Check sheet for the modelled part. Datum: model origin and axes. Units: mm. Face numbers are marked on the shaded views. A direction names the side the tool comes from. Give positions to 0.01 mm unless a question says otherwise; leave off trailing zeros. Order: outer loops, then holes, each group sorted by start corner. A loop starts at its lowest first (then second) coordinate and runs counter-clockwise, first axis right, second up.
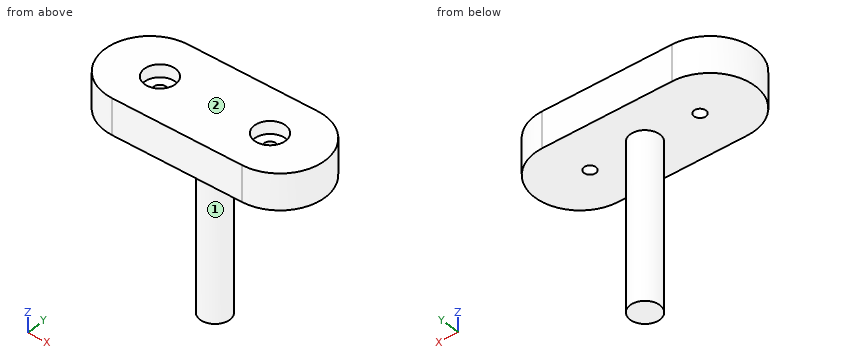
```python
from build123d import *

# Parameters (mm, degrees)
SALIENTE_EXTRUIR1_DEPTH = 9.63
CROQUIS2_R              = 3.98
SALIENTE_EXTRUIR2_DEPTH = 44.5
CROQUIS3_R              = 1.6
CORTAR_EXTRUIR1_DEPTH   = 63.977202423
CROQUIS4_R              = 4.18
CORTAR_EXTRUIR2_DEPTH   = 3.39


with BuildPart() as part:
    # Croquis1 → Saliente-Extruir1 (new body)
    with BuildSketch(Plane.XY):
        with BuildLine():
            Line((-17.685, 12.13), (17.685, 12.13))
            ThreePointArc((17.685, 12.13), (29.815, 0), (17.685, -12.13))
            Line((17.685, -12.13), (-17.685, -12.13))
            ThreePointArc((-17.685, -12.13), (-29.815, 0), (-17.685, 12.13))
        make_face()
    extrude(amount=-SALIENTE_EXTRUIR1_DEPTH)

    # Croquis2 → Saliente-Extruir2 (add)
    with BuildSketch(Plane(origin=(0, 0, -9.63), x_dir=(-1, 0, 0), z_dir=(0, 0, -1))):
        with Locations(Location((0, 0, 0), (0, 0, 180))):
            Circle(CROQUIS2_R)
    extrude(amount=SALIENTE_EXTRUIR2_DEPTH)

    # Croquis3 → Cortar-Extruir1 (cut, through all)
    with BuildSketch(Plane.XY):
        with Locations((-15, 0)):
            Circle(CROQUIS3_R)
        with Locations((15, 0)):
            Circle(CROQUIS3_R)
    extrude(amount=-CORTAR_EXTRUIR1_DEPTH, mode=Mode.SUBTRACT)

    # Croquis4 → Cortar-Extruir2 (cut)
    with BuildSketch(Plane.XY):
        with Locations((-15, 0)):
            Circle(CROQUIS4_R)
        with Locations((15, 0)):
            Circle(CROQUIS4_R)
    extrude(amount=-CORTAR_EXTRUIR2_DEPTH, mode=Mode.SUBTRACT)


solid = part.part
```
(1) Material ranges on L1, parallel to Y at x = -15, z = -8; L2, parallel to Y at x = -15, z = -2; L3, parallel to Z at x = -20, y = 2.75, recorded low to high.
Response values:
L1: y = -12.13 to -1.6, 1.6 to 12.13
L2: y = -12.13 to -4.18, 4.18 to 12.13
L3: z = -9.63 to 0
(2) Cross-section at B-B on y = 0. Enter the section's corners in (x, z) (3 decimals).
Response values:
outline: (-29.815, -9.63) - (-16.6, -9.63) - (-16.6, -3.39) - (-19.18, -3.39) - (-19.18, 0) - (-29.815, 0) - close; (-13.4, -9.63) - (-3.98, -9.63) - (-3.98, -54.13) - (3.98, -54.13) - (3.98, -9.63) - (13.4, -9.63) - (13.4, -3.39) - (10.82, -3.39) - (10.82, 0) - (-10.82, 0) - (-10.82, -3.39) - (-13.4, -3.39) - close; (16.6, -9.63) - (29.815, -9.63) - (29.815, 0) - (19.18, 0) - (19.18, -3.39) - (16.6, -3.39) - close
(3) Set-up check for the marked faces 1 and 2: record each of +Z, -Z, +X, -X, +Y, -Y from which the full face is reachable in a straight line by a thin tool's end or side.
Response values:
face 1: -Z
face 2: +Z, +X, -X, +Y, -Y
(4) Cross-section at A-A on x = -15. Enter the section's corners in (y, z).
Response values:
outline: (-12.13, -9.63) - (-1.6, -9.63) - (-1.6, -3.39) - (-4.18, -3.39) - (-4.18, 0) - (-12.13, 0) - close; (1.6, -9.63) - (12.13, -9.63) - (12.13, 0) - (4.18, 0) - (4.18, -3.39) - (1.6, -3.39) - close
(5) Cross-section at C-C on x = 0. Enter the section's corners in (y, z), then the cut area to 3 significant figures.
Response values:
outline: (-12.13, -9.63) - (-3.98, -9.63) - (-3.98, -54.13) - (3.98, -54.13) - (3.98, -9.63) - (12.13, -9.63) - (12.13, 0) - (-12.13, 0) - close
area: 588 mm2
(6) Cross-section at D-D on z = -11.5. Enter the section's corners in (x, y).
Response values:
outline: circle Ø7.96 at (0, 0)
(7) Gauge pin test, flat ends, axial feed: pin 1 Ø1.5 at (y, z) = (-5, -28) entering from +X; pin 2 Ø3 at (y, z) = (5, -18) entering from -X; pin 3 Ø5 at (x, z) = (-5, -11) entering from -Y; pin 4 Ø8 at (x, z) = (2.5, -32) entering from -Y. Record the tip position at first contact, or that the pin passes through.
Response values:
pin 1: passes through
pin 2: stops at x = -1.89
pin 3: stops at y = -12.13
pin 4: stops at y = -3.98
